Drawing for the job (mm, zero at the part's lowest x, y, z). A direction names the side the tool comes from. Round coordinates to 2 decimals unless told otherwise and drop trailing zeros. Write each loop counter-clockwise with the first axis right and the second up, starting at its lowest first coordinate (ties: lowest second). Pieces come first, ordered by that corner, then holes. Notation, with made-up numbers: (37, 5.5) -> (50, 5.5) arc R24 ccw to (50, 29.5) -> close; hole circle Ø4 at (-4.75, 83). An arc over 180 degrees is marked (long way). One line per question, with ' | ' between items.
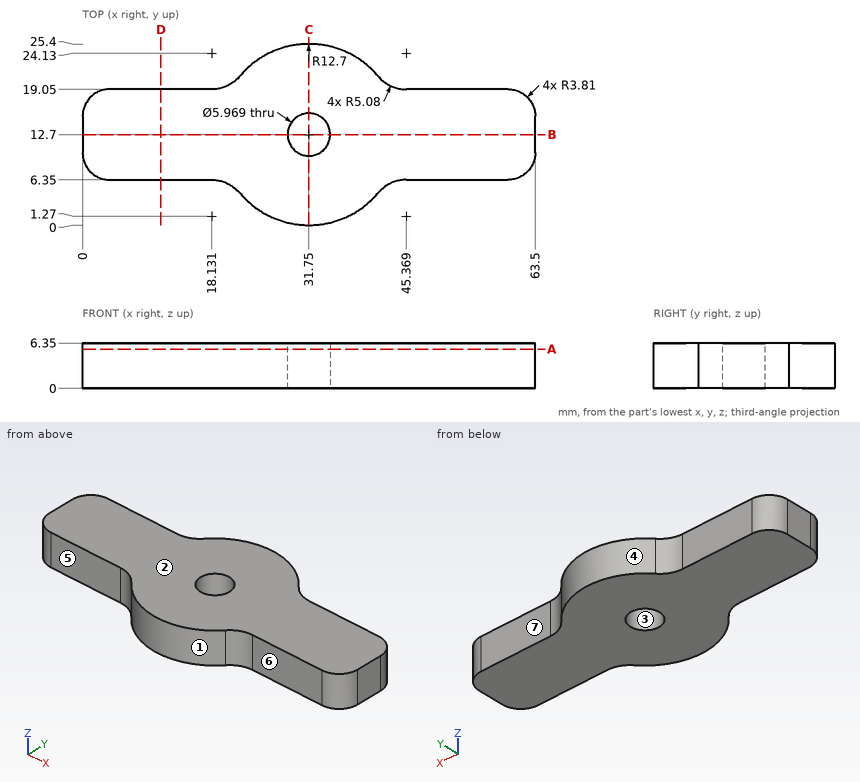
(1) Slice it at B-B (y = 12.7). Write the cut outline in (x, z), then the cut area to 3 significant figures.
Calculated:
outline: (0, 0) -> (28.77, 0) -> (28.77, 6.35) -> (0, 6.35) -> close; (34.73, 0) -> (63.5, 0) -> (63.5, 6.35) -> (34.73, 6.35) -> close | area: 365 mm2
(2) Wall check: line 1 (Y direction, x = 31.75, z = 2); line 2 (Y direction, x = 53, z = 3); line 3 (X direction, y = 15, z = 0.75). Give the ranges that are in metal, low to high. Write a range as from..to.
Calculated:
line 1: 0..9.72, 15.68..25.4 | line 2: 6.35..19.05 | line 3: 0..29.85, 33.65..63.5
(3) Mould opens along Y. For the marked faces 1, 2, 3 and 4 say: pulls with the +Y half, pulls with the -Y half, needs draft (parallel to the pull), parting line crosses it, or undercut.
Calculated:
face 1: pulls with the -Y half | face 2: needs draft | face 3: undercut | face 4: pulls with the +Y half
(4) Drop a flat-ended pin along its axis: pin 1 (3 mm diameter, centred on x = 50, z = 3, fed in from -Y). Give the stop position or say it passes through.
Calculated:
pin 1: y = 6.35
(5) Slice it at A-A (z = 5.5). Write the cut outline in (x, y), then the cut area to 3 significant figures.
Calculated:
outline: (0, 10.16) arc R3.81 ccw to (3.81, 6.35) -> (18.13, 6.35) arc R5.08 cw to (22.02, 4.54) arc R12.7 ccw to (41.48, 4.54) arc R5.08 cw to (45.37, 6.35) -> (59.69, 6.35) arc R3.81 ccw to (63.5, 10.16) -> (63.5, 15.24) arc R3.81 ccw to (59.69, 19.05) -> (45.37, 19.05) arc R5.08 cw to (41.48, 20.86) arc R12.7 ccw to (22.02, 20.86) arc R5.08 cw to (18.13, 19.05) -> (3.81, 19.05) arc R3.81 ccw to (0, 15.24) -> close; hole circle Ø5.97 at (31.75, 12.7) | area: 968 mm2
(6) Slice it at D-D (x = 11). Write the cut outline in (y, z).
Calculated:
outline: (6.35, 0) -> (19.05, 0) -> (19.05, 6.35) -> (6.35, 6.35) -> close
(7) 3-axis set-ups, long thin cutter, end or side, ignore diameter. For the marked faces 5, 6 and 7: which of +Z, -Z, +X, -X, +Y, -Y reach the whole face in a straight line?
Calculated:
face 5: +Z, -Z, -X, -Y | face 6: +Z, -Z, +X, -Y | face 7: +Z, -Z, +X, +Y
(8) Slice it at C-C (x = 31.75). Write the cut outline in (y, z).
Calculated:
outline: (0, 0) -> (9.72, 0) -> (9.72, 6.35) -> (0, 6.35) -> close; (15.68, 0) -> (25.4, 0) -> (25.4, 6.35) -> (15.68, 6.35) -> close
